Design review of the part shown in the three views and the two pictorial views. Dimensions are in mm from the part's minimum x, y and z. A direction names the side the tool comes from. Give positions to 0.01 mm unless a question says otherwise; leave off trailing zeros. Loops run counter-clockwise (first coordinate to the right, second up) from the corner with the lowest first, then second, coordinate; pieces in that order, holes last. Notation, with made-up numbers: (64.5, 48.5) - (119.5, 48.5) arc R36 cw to (119.5, 83.5) - close; hole circle Ø5 at (50, -34). An arc over 180 degrees is marked (long way). Answer in a Markdown table with one row per item.
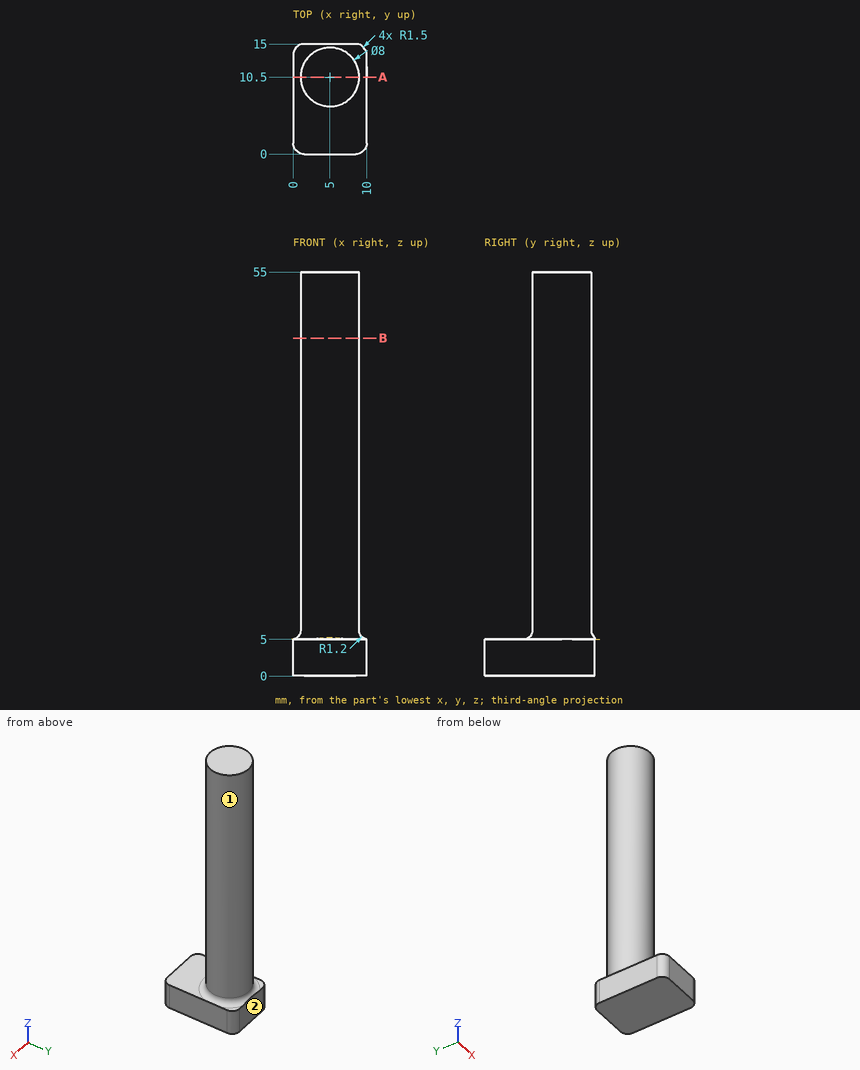
1. We need section A-A, the plane y = 10.5. Give the boundary of the cut face in (x, z).
Values:
| item | result |
|---|---|
| outline | (0, 0) - (10, 0) - (10, 5.02) arc R1.2 cw to (9, 6.2) - (9, 55) - (1, 55) - (1, 6.2) arc R1.2 cw to (0, 5.02) - close |
2. Wall thickness on line 1 (Z direction, x = 5.75, y = 2.5); line 2 (X direction, y = 10.75, z = 18); line 3 (Y direction, x = 4.75, z = 37.5): over which ranges is each line inside the solid? List them lowest first. Write a range as [from, to].
Values:
| item | result |
|---|---|
| line 1 | z = [0, 5] |
| line 2 | x = [1.01, 8.99] |
| line 3 | y = [6.51, 14.49] |
3. Clearance check with flat-ended pins moving along their axes: pin 1 (3 mm diameter, centred on x = 6.5, z = 29, fed in from -Y); pin 2 (1.2 mm diameter, centred on x = 9.5, y = 14, fed in from +Z); pin 3 (6 mm diameter, centred on y = 6, z = 23.5, fed in from -X); pin 4 (5 mm diameter, centred on x = 4, y = 5.5, fed in from +Z). State where each tip first meets the part, or that it passes through.
Values:
| item | result |
|---|---|
| pin 1 | stops at y = 6.5 |
| pin 2 | stops at z = 5 |
| pin 3 | stops at x = 1.29 |
| pin 4 | stops at z = 55 |
4. We need section B-B, the plane z = 46. Give the boundary of the cut face in (x, y), and give its area (3 significant figures).
Values:
| item | result |
|---|---|
| outline | circle Ø8 at (5, 10.5) |
| area | 50.3 mm^2 |
5. For the marked faces 1 and 2, list the 3-axis set-ups (+Z, -Z, +X, -X, +Y, -Y) from which the entire face can be reached by the end or side of a thin tool; tool diameter is ignored.
Values:
| item | result |
|---|---|
| face 1 | +Z |
| face 2 | +Z, -Z, +X, -X, +Y |
